Read the model definition and answer for the solid it produces. Units are mm, in the model's axes. A direction names the side the tool comes from. Coordinates: 2 decimals unless noted, no trailing zeros. Order: outer loops, then holes, each group sorted by start corner. A loop starts at its lowest first (then second) coordinate and runs counter-clockwise, first axis right, second up. Notation, with made-up numbers: (35, 43.5) -> (66, 43.5) arc R18 ccw to (66, 68.5) -> close; hole circle Ø9 at (12.25, 32.25). An arc over 180 degrees is marked (long way). Answer as a JSON object with one key per item and string values. Group by question number.
1) Determine the mould class of faces 1 (the flat face through (7, -13, 0)), 2 (the cylindrical face through (-6, -6, 0)), 3 (the cylindrical face through (0.196, -151.685, 1.201)) for opening direction Z: released by +Z, released by -Z, zero draft, split by the parting line, or undercut.
2) Section A-A on z = 0 is taken. Determine the outline of the cut face in (x, y), and give its area (3 significant figures).
3) Section D-D on z = 8.25 is taken. Determine the outline of the cut face in (x, y).
4) Consider L1, parallel to Y at x = -6.5, z = 0; L2, parallel to Y at x = 6, z = -5; L3, parallel to Z at x = -0.5, y = -155.5. Determine where each line is inside the solid, lowest interval first.
5) Given pin 1 (6 mm diameter, centred on y = -109.5, z = 11, fed in from +X); pin 2 (2 mm diameter, centred on x = 10, y = -150, fed in from +Z); pin 3 (10 mm diameter, centred on y = -35, z = 0, fed in from +X), each flat-ended and moving along its own axis, determine where each tip first touches the part or whether it passes through.
6) A tool of negligible diameter and unlimited length cuts with its end or side. For faces 4 (the flat face through (-3, -143, 10)), 5 (the flat face through (0, -168, 0)), 6 (the flat face through (7, 0, 0)), from which of +Z, -Z, +X, -X, +Y, -Y can it reach the whole face along a straight path? Write none if from no direction.
7) Section C-C on y = -32 is taken. Determine the outline of the cut face in (x, z), and give its area (3 significant figures).
8) Section B-B on x = 0 is taken. Determine the outline of the cut face in (y, z).
Autodesk Fusion 360 part; units mm, degrees
sketch "Sketch1" plane through (0, 0, 0) normal (0, 1, 0) x (1, 0, 0)
  circle A0 centre (0, 0) radius 10
  circle A1 centre (0, 0) radius 6
  dimension "d1" = 20
  dimension "d2" = 12
extrude "Extrude1" add sketch "Sketch1" along normal blind 10 contours A0 | A1
extrude "Extrude3" add sketch "Sketch1" against normal blind 13 contours A1
extrude "Extrude4" add sketch "Sketch1" against normal blind 130 from surface at -13 contours A0 | A1
sketch "Sketch2" plane through (0, -143, 0) normal (0, -1, 0) x (1, 0, 0)
  circle A0 centre (0, 0) radius 10
  circle A1 centre (0, 0) radius 14
  dimension "d12" = 28
extrude "Extrude5" add sketch "Sketch2" along normal blind 25 contours A0 | A1
thread "Thread1"
sketch "Sketch3" plane through (0, 0, 0) normal (1, 0, 0) x (0, 1, 0)
  circle A0 centre (-155.5, 0) radius 4
  line L0 (-143, 14) -> (-143, -14)
  dimension "d15" = 8
  dimension "d20" = 12.5
extrude "Extrude6" cut sketch "Sketch3" along normal up to surface and the other way blind 14 end surface at (13.9304, -151.3333, -1.3939)
Worked answers:
{
 "1": {"face 1": "zero draft", "face 2": "split by the parting line", "face 3": "undercut"},
 "2": {"outline": "(-14, -168) -> (14, -168) -> (14, -159.5) -> (-14, -159.5) -> close; (-14, -151.5) -> (14, -151.5) -> (14, -143) -> (10, -143) -> (10, -13) -> (6, -13) -> (6, 0) -> (10, 0) -> (10, 10) -> (-10, 10) -> (-10, 0) -> (-6, 0) -> (-6, -13) -> (-10, -13) -> (-10, -143) -> (-14, -143) -> close", "area": "3,430 mm²"},
 "3": {"outline": "(-11.31, -168) -> (11.31, -168) -> (11.31, -143) -> (5.65, -143) -> (5.65, -13) -> (-5.65, -13) -> (-5.65, -143) -> (-11.31, -143) -> close; (-5.65, 0) -> (5.65, 0) -> (5.65, 10) -> (-5.65, 10) -> close"},
 "4": {"L1": "y = -168 to -159.5, -151.5 to -13, 0 to 10", "L2": "y = -168 to -13, 0 to 10", "L3": "z = -13.99 to -4, 4 to 13.99"},
 "5": {"pin 1": "stops at x = 6", "pin 2": "stops at z = 10.72", "pin 3": "stops at x = 10"},
 "6": {"face 4": "+Y", "face 5": "+Z, -Z, +X, -X, -Y", "face 6": "none"},
 "7": {"outline": "circle Ø20 at (0, 0)", "area": "314 mm²"},
 "8": {"outline": "(-168, -14) -> (-143, -14) -> (-143, -10) -> (-13, -10) -> (-13, -6) -> (0, -6) -> (0, -10) -> (10, -10) -> (10, 10) -> (0, 10) -> (0, 6) -> (-13, 6) -> (-13, 10) -> (-143, 10) -> (-143, 14) -> (-168, 14) -> close; hole circle Ø8 at (-155.5, 0)"}
}
